Geometry: final body of the model. Coordinates: model frame, mm. Face numbers are marked on the shaded views. Give positions to 0.01 mm unless a question says otherwise; leave off trailing zeros. Order: outer loops, then holes, each group sorted by start corner. A loop starts at its lowest first (then second) coordinate and runs counter-clockwise, first axis right, second up. Notation, with made-up numbers: M -13.5,22 L 2.5,22 A32 cw 2.5,52 Z; hole C 1.25,-25.75 d3. An arc over 180 degrees is marked long. One line per item, written item: value. Start each with the question number.
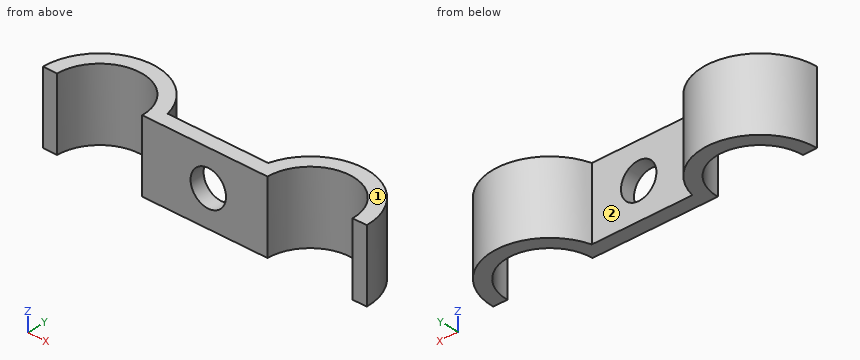
```python
from build123d import *

# Parameters (mm, degrees)
Y_KSEKLIK_EKSTR_ZYON1_DEPTH = 10
KES_EKSTR_ZYON1_DEPTH       = 10
KES_EKSTR_ZYON1_DEPTH_BACK  = 5
IZIM2_R                     = 2.5


with BuildPart() as part:
    # Çizim1 → Yükseklik-Ekstrüzyon1 (new body)
    with BuildSketch(Plane.XY):
        with BuildLine():
            Line((0, 0), (17.68, 0))
            ThreePointArc((17.68, 0), (23.68, 6), (29.68, 0))
            Line((29.68, 0), (31.68, 0))
            ThreePointArc((31.68, 0), (24.68803434, 7.93623757), (15.934033308, 2))
            Line((15.934033308, 2), (1.745966692, 2))
            ThreePointArc((1.745966692, 2), (-7.00803434, 7.93623757), (-14, 0))
            Line((-14, 0), (-12, 0))
            ThreePointArc((-12, 0), (-6, 6), (0, 0))
        make_face()
    extrude(amount=Y_KSEKLIK_EKSTR_ZYON1_DEPTH)

    # Çizim2 → Kes-Ekstrüzyon1 (cut, two sides: drawn at the far end of the back side and taken through both)
    with BuildSketch(Plane(origin=(0, 2, 0), x_dir=(1, 0, 0), z_dir=(0, 1, 0)).offset(-KES_EKSTR_ZYON1_DEPTH_BACK)):
        with Locations((9.316, -5)):
            Circle(IZIM2_R)
    extrude(amount=KES_EKSTR_ZYON1_DEPTH + KES_EKSTR_ZYON1_DEPTH_BACK, mode=Mode.SUBTRACT)


solid = part.part
```
Q1. Section query D-D on x = -6. Return loops of the section in (y, z).
Q2. Section query B-B on z = 1.5. Return loops of the section in (x, y), and give its area (3 significant figures).
Q3. Ray query, line 1 along X through (y, z) = (5.5, 5.25); line 2 along X through (y, z) = (2.5, 7); line 3 along X through (y, z) = (7, 1.5). Return the intervals inside material, ascending. Write a range as [from, to].
Q4. Contact query for a flat-ended pin moving along its axis: pin 1 (6 mm diameter, centred on x = 12.5, z = 5, fed in from +Y). Output: stop coordinate, or through.
Q5. Section query C-C on y = 6.75. Return loops of the section in (x, z), and give its area (3 significant figures).
Q6. Section query A-A on z = 5. Return loops of the section in (x, y), and give its area (3 significant figures).
Q7. Mould query, pull axis X, two halves, no side actions, for the marked faces 1 and 2. Classes: +X half, -X half, draft (parallel to the pull), parting line (faces both ways), or undercut.
Results below:
1. outline: M 6,0 L 8,0 L 8,10 L 6,10 Z
2. outline: M -14,0 L -12,0 A6 cw 0,0 L 17.68,0 A6 cw 29.68,0 L 31.68,0 A8 ccw 15.93,2 L 1.75,2 A8 ccw Z
2. area: 116 mm2
3. line 1: [-11.81, -8.4], [-3.6, -0.19], [17.87, 21.28], [26.08, 29.49]
3. line 2: [-13.6, -11.45], [-0.55, 1.6], [16.08, 18.23], [29.13, 31.28]
3. line 3: [-9.87, -2.13], [19.81, 27.55]
4. pin 1: y = 2
5. outline: M -10.29,0 L -1.71,0 L -1.71,10 L -10.29,10 Z; M 19.39,0 L 27.97,0 L 27.97,10 L 19.39,10 Z
5. area: 172 mm2
6. outline: M -14,0 L -12,0 A6 cw 0,0 L 6.82,0 L 6.82,2 L 1.75,2 A8 ccw Z; M 11.82,0 L 17.68,0 A6 cw 29.68,0 L 31.68,0 A8 ccw 15.93,2 L 11.82,2 Z
6. area: 106 mm2
7. face 1: draft
7. face 2: undercut
